Check sheet for the modelled part. Datum: model origin and axes. Units: mm. A direction names the side the tool comes from. Give positions to 0.01 mm unless a question says otherwise; leave off trailing zeros. Loops run counter-clockwise (first coordinate to the right, second up) from the corner with the lowest first, then second, coordinate; pieces in that order, holes last. Notation, with made-up numbers: (-36.5, 2) - (-1.5, 2) arc R15 cw to (-1.5, 7) - close; hole circle Ø10 at (-35.75, 51.5). An arc over 180 degrees is marked (long way). Answer in a Markdown table with one row per item. Add a question column.
(1) Set-up check for faces 4 (the face through (8, 10, 8)), 5 (the face through (-4, 2, 6)), 6 (the face through (21, 6, 1.25)): record each of +Z, -Z, +X, -X, +Y, -Y from which the full face is reachable in a straight line by a thin tool's end or side.
(2) Sectioned sample at D-D on x = 3. Enter the section's corners in (y, z).
(3) Draft check along X on faces 1 (the face through (8, 14, 1)), 2 (the face through (17.592, 15.293, 15.859)), 3 (the face through (0.74, 29.22, 10.98)). Enter one of: released by +X, released by -X, zero draft, split by the parting line, or undercut.
(4) Sectioned sample at A-A on x = 9. Enter the section's corners in (y, z), then the cut area to 3 significant figures.
(5) Thickness scan on L1, parallel to Y at x = 0.5, z = 8.5; L2, parallel to X at y = 33, z = 13.5. Record the ranges inside material, lowest first.
(6) Go/stop test with flat-tipped pins: P1, Ø3, axis at x = 20, z = 10, coming from the +Y side; P2, Ø1.5, axis at y = 32, z = 11, coming from the +X side; P3, Ø6, axis at y = 30, z = 8.5, coming from the -X side. Record where each tip stops, or that it passes through.
(7) Sectioned sample at C-C on z = 13.75. Enter the section's corners in (x, y).
(8) Sectioned sample at B-B on y = 15. Enter the section's corners in (x, z).
from build123d import *

# Parameters (mm, degrees)
BASE_SHAPE_DEPTH      = 17
SKETCH2_W             = 14
SKETCH2_H             = 14
CENTER_SLOT_DEPTH     = 27
SKETCH4_W             = 10
SKETCH4_H             = 13.5
WING_CUT_OUTS_DEPTH   = 16.5
SKETCH5_R             = 1.75
WING_HOLES_DEPTH      = 48.360320945
WIRE_SLOT_REACH       = 50.857
SKETCH6_W             = 5
SKETCH6_H             = 2
LOAD_CELL_HOLES_REACH = 50.857
SKETCH7_R             = 2.6


with BuildPart() as part:
    # Sketch1 → Base Shape (new body)
    with BuildSketch(Plane.XY):
        with BuildLine():
            Line((0, 18.313708499), (0, 37))
            Line((0, 37), (17, 37))
            Line((17, 37), (17, 18.313708499))
            ThreePointArc((17, 18.313708499), (17.60896374, 15.25224104), (19.343145751, 12.656854249))
            Line((19.343145751, 12.656854249), (27, 5))
            Line((27, 5), (27, 0))
            Line((27, 0), (17, 0))
            Line((17, 0), (0, 0))
            Line((0, 0), (-10, 0))
            Line((-10, 0), (-10, 5))
            Line((-10, 5), (-2.343145751, 12.656854249))
            ThreePointArc((-2.343145751, 12.656854249), (-0.60896374, 15.25224104), (0, 18.313708499))
        make_face()
    extrude(amount=BASE_SHAPE_DEPTH)

    # Sketch2 → Center Slot (cut)
    with BuildSketch(Plane(origin=(0, 37, 0), x_dir=(1, 0, 0), z_dir=(0, 1, 0))):
        with Locations((8.5, -8.5)):
            Rectangle(SKETCH2_W, SKETCH2_H)
    extrude(amount=-CENTER_SLOT_DEPTH, mode=Mode.SUBTRACT)

    # Sketch4 → Wing Cut Outs (cut)
    with BuildSketch(Plane(origin=(0, 2, 0), x_dir=(-1, 0, 0), z_dir=(0, -1, 0))):
        with Locations((5, -8)):
            Rectangle(SKETCH4_W, SKETCH4_H)
    wing_cut_outs = extrude(amount=-WING_CUT_OUTS_DEPTH, mode=Mode.SUBTRACT)

    # Mirror1: Wing Cut Outs across plane
    add(wing_cut_outs.mirror(Plane(origin=(8.5, 0, 0), x_dir=(0, 0, 1), z_dir=(1, 0, 0))), mode=Mode.SUBTRACT)

    # Sketch5 → Wing Holes (cut, through all)
    with BuildSketch(Plane(origin=(0, 2, 0), x_dir=(-1, 0, 0), z_dir=(0, -1, 0))):
        with Locations(Location((5, -8, 0), (0, 0, 180))):
            Circle(SKETCH5_R)
    wing_holes = extrude(amount=WING_HOLES_DEPTH, mode=Mode.SUBTRACT)

    # Mirror2: Wing Holes across plane
    add(wing_holes.mirror(Plane(origin=(8.5, 0, 0), x_dir=(0, 0, 1), z_dir=(1, 0, 0))), mode=Mode.SUBTRACT)

    # Sketch6 → Wire Slot (cut, up to next)
    with BuildSketch(Plane.XY, mode=Mode.PRIVATE) as wire_slot_sk1:
        with Locations((8, 15)):
            Rectangle(SKETCH6_W, SKETCH6_H)
    wire_slot_tool1 = extrude(wire_slot_sk1.sketch, amount=WIRE_SLOT_REACH, mode=Mode.PRIVATE) & part.part
    add(wire_slot_tool1.solids().sort_by_distance((8, 15, 0))[0], mode=Mode.SUBTRACT)

    # Sketch7 → Load Cell Holes (cut, up to next)
    with BuildSketch(Plane(origin=(0, 0, 0), x_dir=(0, 0, -1), z_dir=(1, 0, 0)), mode=Mode.PRIVATE) as load_cell_holes_sk1:
        with Locations(Location((-8.5, 15, 0), (0, 0, 180))):
            Circle(SKETCH7_R)
    load_cell_holes_tool1 = extrude(load_cell_holes_sk1.sketch, amount=LOAD_CELL_HOLES_REACH, mode=Mode.PRIVATE) & part.part
    # Sketch7 → Load Cell Holes (cut, up to next)
    with BuildSketch(Plane(origin=(0, 0, 0), x_dir=(0, 0, -1), z_dir=(1, 0, 0)), mode=Mode.PRIVATE) as load_cell_holes_sk2:
        with Locations(Location((-8.5, 30, 0), (0, 0, 180))):
            Circle(SKETCH7_R)
    load_cell_holes_tool2 = extrude(load_cell_holes_sk2.sketch, amount=LOAD_CELL_HOLES_REACH, mode=Mode.PRIVATE) & part.part
    load_cell_holes_1 = load_cell_holes_tool1.solids().sort_by_distance((0, 15, 8.5))[0]
    add(load_cell_holes_1, mode=Mode.SUBTRACT)
    load_cell_holes_2 = load_cell_holes_tool2.solids().sort_by_distance((0, 30, 8.5))[0]
    add(load_cell_holes_2, mode=Mode.SUBTRACT)
    load_cell_holes = load_cell_holes_1 + load_cell_holes_2  # Load Cell Holes as one shape, for the pattern or mirror that repeats it

    # Mirror3: Load Cell Holes across plane
    add(load_cell_holes.mirror(Plane(origin=(8.5, 0, 0), x_dir=(0, 0, 1), z_dir=(1, 0, 0))), mode=Mode.SUBTRACT)


solid = part.part
Reply:
| question | item | result |
|---|---|---|
| 1 | face 4 | +Y |
| 1 | face 5 | -X, +Y |
| 1 | face 6 | +X, +Y |
| 2 | outline | (0, 0) - (37, 0) - (37, 1.5) - (10, 1.5) - (10, 15.5) - (37, 15.5) - (37, 17) - (0, 17) - close |
| 3 | face 1 | undercut |
| 3 | face 2 | released by +X |
| 3 | face 3 | zero draft |
| 4 | outline | (0, 0) - (14, 0) - (14, 1.5) - (10, 1.5) - (10, 15.5) - (37, 15.5) - (37, 17) - (0, 17) - close; (16, 0) - (37, 0) - (37, 1.5) - (16, 1.5) - close |
| 4 | area | 248 mm^2 |
| 5 | L1 | 0 to 12.4, 17.6 to 27.4, 32.6 to 37 |
| 5 | L2 | 0 to 1.5, 15.5 to 17 |
| 6 | P1 | y = 2 |
| 6 | P2 | x = 17 |
| 6 | P3 | x = 0 |
| 7 | outline | (-10, 0) - (27, 0) - (27, 2) - (17, 2) - (17, 37) - (15.5, 37) - (15.5, 10) - (1.5, 10) - (1.5, 37) - (0, 37) - (0, 2) - (-10, 2) - close |
| 8 | outline | (-0.72, 0) - (5.5, 0) - (5.5, 1.5) - (1.5, 1.5) - (1.5, 5.9) - (0, 5.9) - (0, 1.25) - (-0.72, 1.25) - close; (-0.72, 14.75) - (0, 14.75) - (0, 11.1) - (1.5, 11.1) - (1.5, 15.5) - (15.5, 15.5) - (15.5, 11.1) - (17, 11.1) - (17, 14.75) - (17.72, 14.75) - (17.72, 17) - (-0.72, 17) - close; (10.5, 0) - (17.72, 0) - (17.72, 1.25) - (17, 1.25) - (17, 5.9) - (15.5, 5.9) - (15.5, 1.5) - (10.5, 1.5) - close |
